Source: CAD feature listing. Evaluate the final solid. Frame: model axes, mm. A direction names the side the tool comes from. Give positions to 0.01 mm unless a question says otherwise; leave off trailing zeros. Order: outer loops, then holes, each group sorted by start corner. A loop starts at its lowest first (then second) coordinate and runs counter-clockwise, first axis right, second up. Notation, with made-up numbers: M 86.25,67.25 L 123.25,67.25 A19 cw 123.25,80.25 Z; hole C -14,48 d1. An arc over 180 degrees is marked long. Answer in a Markdown table with one row per item. Add a question column.
(1) Section query B-B, the plane y = -10.5. Return loops of the section in (x, z), plus the area to 3 significant figures.
(2) Set-up query: faces 1 (the face through (18, 19, 74.8)), 2 (the face through (9.247, -17, 8)), 3 (the face through (-21, -14, 26.716)). Return all of +Z, -Z, +X, -X, +Y, -Y with unobstructed straight access to the full face (end or side cutting, diameter ignored); none if empty.
(3) Material intervals for line 1 along X through (y, z) = (13, 66); line 2 along Z through (x, y) = (4.5, 6); line 3 along Z through (x, y) = (-29, -13), sorted ascending.
(4) Mould query, pull axis Y, two halves, no side actions, for faces 4 (the face through (-11.773, -14, 34)), 5 (the face through (14.088, 9.858, 61.933)), 6 (the face through (18, 13, 48.7)), 7 (the face through (7, -14.714, 7)). Classes: pulls with the +Y half, pulls with the -Y half, needs draft (parallel to the pull), parting line crosses it, or undercut.
(5) Section query D-D, the plane z = 40. Return loops of the section in (x, y).
(6) Section query C-C, the plane y = 9. Return loops of the section in (x, z), plus the area to 3 significant figures.
(7) Section query A-A, the plane z = 10. Return loops of the section in (x, y).
(8) Pin query (flat end, axial travel): P1, Ø1, axis at x = -18, y = 15.5, coming from the +Z side; P2, Ø6, axis at x = -27.5, y = 17.5, coming from the -Z side; P3, Ø0.9, axis at x = 7.5, z = 7.5, coming from the -Y side; P4, Ø5.5, axis at x = 5.5, y = -17.5, coming from the -Z side. Return the tip coordinate at first contact, or that it passes through.
from build123d import *

# Parameters (mm, degrees)
F0_W      = 70.3775063157
F0_H      = 41.7411420494
F1_DEPTH  = 49.8
F2_W      = 9.2471539974
F2_H      = 15.9300006926
F3_DEPTH  = 5
F4_W      = 18.7503434718
F4_H      = 14.2625961453
F4_W_2    = 21.2060459889
F4_H_2    = 14.3702477217
F5_DEPTH  = 10
F6_R      = 7.2844766826
F7_DEPTH  = 25
F8_R      = 5.3356487736
F9_DEPTH  = 26.1
F10_R     = 0.9417381486
F11_DEPTH = 0.3


with BuildPart() as f1:
    # F0 (on Top) → F1 (new body)
    with BuildSketch(Plane.XY):
        with Locations((-0.606700778, 1.4560865238)):
            Rectangle(F0_W, F0_H)
    extrude(amount=F1_DEPTH)

    # F2 (on face) → F3 (cut)
    with BuildSketch(Plane.XZ.offset(19.4144845009)):
        with Locations((4.6235769987, 7.9650003463)):
            Rectangle(F2_W, F2_H)
    extrude(amount=-F3_DEPTH, mode=Mode.SUBTRACT)

    # F4 (on face) → F5 (cut)
    with BuildSketch(Plane.XZ.offset(19.4144845009)):
        with Locations((-21.1479142308, 33.8475396857)):
            Rectangle(F4_W, F4_H)
        with Locations((16.3835778367, 33.7937138975)):
            Rectangle(F4_W_2, F4_H_2)
    extrude(amount=-F5_DEPTH, mode=Mode.SUBTRACT)

    # F6 (on face) → F7 (join)
    with BuildSketch(Plane.XY.offset(49.8)):
        with Locations((18.3224212378, 13.1047777832)):
            Circle(F6_R)
    extrude(amount=F7_DEPTH)

    # F8 (on face) → F9 (cut)
    with BuildSketch(Plane.XY.offset(74.8)):
        with Locations((18.3224212378, 13.1047777832)):
            Circle(F8_R)
    extrude(amount=-F9_DEPTH, mode=Mode.SUBTRACT)

    # F10 (on face) → F11 (join)
    with BuildSketch(Plane.XZ.offset(14.4144845009)):
        with Locations((7.1194134653, 7.4219265953)):
            Circle(F10_R)
    extrude(amount=F11_DEPTH)


solid = f1.part
Values follow:
| question | item | result |
|---|---|---|
| 1 | outline | M -35.8,0 L 34.58,0 L 34.58,49.8 L -35.8,49.8 Z; hole M -30.52,26.72 L -11.77,26.72 L -11.77,40.98 L -30.52,40.98 Z; hole M 5.78,26.61 L 26.99,26.61 L 26.99,40.98 L 5.78,40.98 Z |
| 1 | area | 2,930 mm² |
| 2 | face 1 | +Z, +X, -X, +Y, -Y |
| 2 | face 2 | -Z, -Y |
| 2 | face 3 | -Y |
| 3 | line 1 | x = 11.04 to 12.99, 23.66 to 25.61 |
| 3 | line 2 | z = 0 to 49.8 |
| 3 | line 3 | z = 0 to 26.72, 40.98 to 49.8 |
| 4 | face 4 | needs draft |
| 4 | face 5 | undercut |
| 4 | face 6 | undercut |
| 4 | face 7 | pulls with the -Y half |
| 5 | outline | M -35.8,-19.41 L -30.52,-19.41 L -30.52,-9.41 L -11.77,-9.41 L -11.77,-19.41 L 5.78,-19.41 L 5.78,-9.41 L 26.99,-9.41 L 26.99,-19.41 L 34.58,-19.41 L 34.58,22.33 L -35.8,22.33 Z |
| 6 | outline | M -35.8,0 L 34.58,0 L 34.58,49.8 L 24.34,49.8 L 24.34,74.8 L 21.73,74.8 L 21.73,48.7 L 14.91,48.7 L 14.91,74.8 L 12.3,74.8 L 12.3,49.8 L -35.8,49.8 Z |
| 6 | area | 3,630 mm² |
| 7 | outline | M -35.8,-19.41 L 0,-19.41 L 0,-14.41 L 9.25,-14.41 L 9.25,-19.41 L 34.58,-19.41 L 34.58,22.33 L -35.8,22.33 Z |
| 8 | P1 | stops at z = 49.8 |
| 8 | P2 | stops at z = 0 |
| 8 | P3 | stops at y = -14.71 |
| 8 | P4 | stops at z = 15.93 |
